Verification items for the finished model (mm, model axes). Face numbers are marked on the shaded views. A direction names the side the tool comes from. Give positions to 0.01 mm unless a question says otherwise; leave off trailing zeros. Order: outer loops, then holes, each group sorted by start corner. A loop starts at its lowest first (then second) coordinate and runs counter-clockwise, first axis right, second up.
(1) Access from +Z, -Z, +X, -X, +Y, -Y to the whole of each face (thin tool, end or side, straight path). Record for the marked faces 4 and 5.
(2) Mould release check, pull along X, two halves, no side actions. Record for the marked faces 1, 2 and 3: pulls with the +X half, pulls with the -X half, needs draft (parallel to the pull), parting line crosses it, or undercut.
(3) Scan lines: L1, parallel to X at y = 36, z = 48.5; L2, parallel to Z at x = 55.5, y = 16; L3, parallel to Y at x = -26.5, z = 57.5. Record each from-to range of solid material in increasing order.
(4) Gauge pin test, flat ends, axial feed: pin 1 (6 mm diameter, centred on y = 18, z = 92.5, fed in from +X); pin 2 (5 mm diameter, centred on y = 68.5, z = 46.5, fed in from -X); pin 3 (10 mm diameter, centred on x = 52.5, z = 30.5, fed in from +Y). Record the tip position at first contact, or that the pin passes through.
(5) Sectioned sample at A-A on z = 74. Record the cut outline in (x, y) (3 decimals).
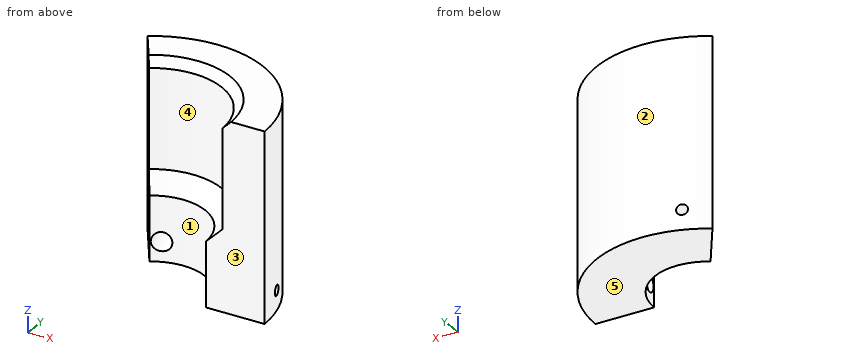
```python
from build123d import *

# Parameters (mm, degrees)
F1_DEPTH  = 143.66875
F7_R      = 3.96875
F8_DEPTH  = 76.2
F6_R      = 7.14375
F9_DEPTH  = 28.575
F11_R     = 7.14375
F13_DEPTH = 28.575
F12_R     = 3.96875
F14_DEPTH = 76.2


with BuildPart() as f1:
    # F0 (on Top) → F1 (new body)
    with BuildSketch(Plane.XY):
        with BuildLine():
            ThreePointArc((-21.784028, 35.058262), (20.056045, 36.074654), (41.275, 0))
            Line((41.275, 0), (85.725, 0))
            ThreePointArc((85.725, 0), (41.654863, 74.924282), (-45.24375, 72.813314))
            Line((-45.24375, 72.813314), (-21.784028, 35.058262))
        make_face()
    extrude(amount=F1_DEPTH)

    # F2 (on face) → F4 (revolve, cut)
    with BuildSketch(Plane(origin=(0, 0, 0), x_dir=(0.527778, -0.849382, 0), z_dir=(-0.849382, -0.527778, 0))):
        Polygon((-53.975, 61.9125), (-41.275, 49.2125), (-41.275, 143.66875), (-60.325, 143.66875), (-53.975, 137.31875), align=None)
    revolve(axis=Axis((0, 0, 45.690566), (0, 0, 1)), mode=Mode.SUBTRACT)

    # F7 (on face) → F8 (cut)
    with BuildSketch(Plane(origin=(-11.304252, 38.162514, 0), x_dir=(-0.95882, -0.284015, 0), z_dir=(-0.284015, 0.95882, 0))):
        with Locations((2.992371, 15.08125)):
            Circle(F7_R)
    extrude(amount=F8_DEPTH, mode=Mode.SUBTRACT)

    # F6 (on face) → F9 (cut)
    with BuildSketch(Plane(origin=(-11.304252, 38.162514, 0), x_dir=(-0.95882, -0.284015, 0), z_dir=(-0.284015, 0.95882, 0))):
        with Locations((2.992371, 15.08125)):
            Circle(F6_R)
    extrude(amount=F9_DEPTH, mode=Mode.SUBTRACT)

    # F11 (on face) → F13 (cut)
    with BuildSketch(Plane(origin=(38.419372, 10.474323, 0), x_dir=(0.263031, -0.964787, 0), z_dir=(-0.964787, -0.263031, 0))):
        with Locations((2.919113, 15.08125)):
            Circle(F11_R)
    extrude(amount=-F13_DEPTH, mode=Mode.SUBTRACT)

    # F12 (on face) → F14 (cut)
    with BuildSketch(Plane(origin=(38.419372, 10.474323, 0), x_dir=(0.263031, -0.964787, 0), z_dir=(-0.964787, -0.263031, 0))):
        with Locations((2.919113, 15.08125)):
            Circle(F12_R)
    extrude(amount=-F14_DEPTH, mode=Mode.SUBTRACT)


solid = f1.part
```
Ans:
1. face 4: +Z, -Y
1. face 5: -Z, +X, -X, +Y, -Y
2. face 1: undercut
2. face 2: parting line crosses it
2. face 3: needs draft
3. L1: x = -22.37 to -20.19, 20.19 to 77.8
3. L2: z = 0 to 9.01, 21.16 to 141.1
3. L3: y = 42.65 to 81.53
4. pin 1: stops at x = 84.4
4. pin 2: stops at x = -44.12
4. pin 3: stops at y = 71.36
5. outline: (-45.244, 72.813) - (-28.487, 45.845) arc R53.975 cw to (53.975, 0) - (85.725, 0) arc R85.725 ccw to start
